from build123d import *

# Parameters (mm, degrees)
F0_W      = 111.730128
F0_H      = 100.016385
F1_DEPTH  = 78.232
F2_W      = 40.233598
F2_H      = 34.137598
F3_DEPTH  = 32.766
F4_R      = 11.566348
F5_DEPTH  = 36.322
F6_R      = 8.876558
F7_DEPTH  = 21.082
F8_W      = 53.551454
F8_H      = 53.157688
F9_DEPTH  = 38.862
F9_FACE_W = 53.551454
F9_FACE_H = 53.157688
F10_DEPTH = 59.944
F12_DEPTH = 31.75


with BuildPart() as f1:
    # F0 (on Top) → F1 (new body)
    with BuildSketch(Plane.XY):
        with Locations((-0.595264, 16.872793)):
            Rectangle(F0_W, F0_H)
    extrude(amount=F1_DEPTH)

    # F2 (on face) → F3 (join)
    with BuildSketch(Plane.XZ.offset(33.135399)):
        with Locations((27.2796, 32.562797)):
            Rectangle(F2_W, F2_H)
    extrude(amount=F3_DEPTH)

    # F4 (on face) → F5 (join)
    with BuildSketch(Plane.XZ.offset(65.901399)):
        with Locations((24.922676, 31.953197)):
            Circle(F4_R)
    extrude(amount=F5_DEPTH)

    # F6 (on face) → F7 (join)
    with BuildSketch(Plane.XZ.offset(102.223399)):
        with Locations((24.922676, 31.953197)):
            Circle(F6_R)
    extrude(amount=F7_DEPTH)

    # F8 (on face) → F9 (join)
    with BuildSketch(Plane.XY.offset(78.232)):
        with Locations((18.703634, 15.429604)):
            Rectangle(F8_W, F8_H)
    extrude(amount=F9_DEPTH)

    # F9_face (on face) → F10 (join)
    with BuildSketch(Plane(origin=(18.703634, 15.429604, 117.094), x_dir=(1, 0, 0), z_dir=(0, 0, 1))):
        Rectangle(F9_FACE_W, F9_FACE_H)
    extrude(amount=F10_DEPTH)

    # F11 (on face) → F12 (join)
    with BuildSketch(Plane.XZ.offset(11.14924)):
        Polygon((25.2405, 142.392326), (25.2405, 155.871343), (14.70218, 164.275372), (1.561111, 161.276009), (-4.287215, 149.131835), (1.561111, 136.98766), (14.70218, 133.988297), align=None)
    extrude(amount=F12_DEPTH)


solid = f1.part
Read the model definition and answer for the solid it produces. Units are mm, in the model's axes. A direction names the side the tool comes from. Round coordinates to 2 decimals unless told otherwise and drop trailing zeros. Write each loop counter-clockwise with the first axis right and the second up, starting at its lowest first coordinate (ties: lowest second). Pieces come first, ordered by that corner, then holes.
1. The part is cut by section D-D, the plane y = -58. Determine the outline of the cut face in (x, z).
2. Determine the mould class of faces 1 (the face through (25, -123.305, 32)), 2 (the face through (-1, 18, 0)), 3 (the face through (18, -11.149, 127)), 4 (the face through (16.055, -112.617, 32.343)) for opening direction Z: pulls with the +Z half, pulls with the -Z half, needs draft (parallel to the pull), parting line crosses it, or undercut.
3. The part is cut by section C-C, the plane x = 31. Determine the outline of the cut face in (y, z).
4. Given pin 1 Ø4 at (x, y) = (2.5, -46) entering from +Z; pin 2 Ø16 at (x, z) = (14.5, 146.5) entering from -Y; pin 3 Ø16 at (y, z) = (4.5, 117.5) entering from +X; pin 4 Ø10 at (x, y) = (35, -60) entering from -Z, each flat-ended and moving along its own axis, determine where each tip first touches the part or whether it passes through.
5. The part is cut by section B-B, the plane z = 94.5. Determine the outline of the cut face in (x, y).
6. Straight lines are drawn through the part: L1, parallel to Y at x = 6.5, z = 131; L2, parallel to X at y = 21, z = 163; L3, parallel to Z at x = -13.5, y = 0. For each, find the intervals that lie inside material, in ascending order.
7. Which of the six approach directions +Z, -Z, +X, -X, +Y, -Y give full straight-line access (tool end or side, diameter ignored) to faces 5 (the face through (10, -42.899, 149)), 6 (the face through (18, 42.008, 127)), 7 (the face through (47.396, -49, 32)), 8 (the face through (-1.32, -26.8, 155.29)), 9 (the face through (23.42, -83.81, 43.42))?
8. The part is cut by section A-A, the plane y = -23. Determine the outline of the cut face in (x, z), then the cut area to 3 significant figures.
Values:
1. outline: (7.16, 15.49) - (47.4, 15.49) - (47.4, 49.63) - (7.16, 49.63) - close
2. face 1: needs draft
2. face 2: pulls with the -Z half
2. face 3: undercut
2. face 4: parting line crosses it
3. outline: (-123.31, 25.48) - (-102.22, 25.48) - (-102.22, 22.11) - (-65.9, 22.11) - (-65.9, 15.49) - (-33.14, 15.49) - (-33.14, 0) - (66.88, 0) - (66.88, 78.23) - (42.01, 78.23) - (42.01, 177.04) - (-11.15, 177.04) - (-11.15, 78.23) - (-33.14, 78.23) - (-33.14, 49.63) - (-65.9, 49.63) - (-65.9, 41.79) - (-102.22, 41.79) - (-102.22, 38.42) - (-123.31, 38.42) - close
4. pin 1: passes through
4. pin 2: stops at y = -42.9
4. pin 3: stops at x = 45.48
4. pin 4: stops at z = 15.49
5. outline: (-8.07, -11.15) - (45.48, -11.15) - (45.48, 42.01) - (-8.07, 42.01) - close
6. L1: y = -11.15 to 42.01
6. L2: x = -8.07 to 45.48
6. L3: z = 0 to 78.23
7. face 5: +Z, +X, -X, -Y
7. face 6: +Z, +X, -X, +Y
7. face 7: +Z, -Z, +X, -Y
7. face 8: +Z, -X, -Y
7. face 9: -Y
8. outline: (-56.46, 0) - (55.27, 0) - (55.27, 78.23) - (-56.46, 78.23) - close; (-4.29, 149.13) - (1.56, 136.99) - (14.7, 133.99) - (25.24, 142.39) - (25.24, 155.87) - (14.7, 164.28) - (1.56, 161.28) - close
8. area: 9,400 mm2
